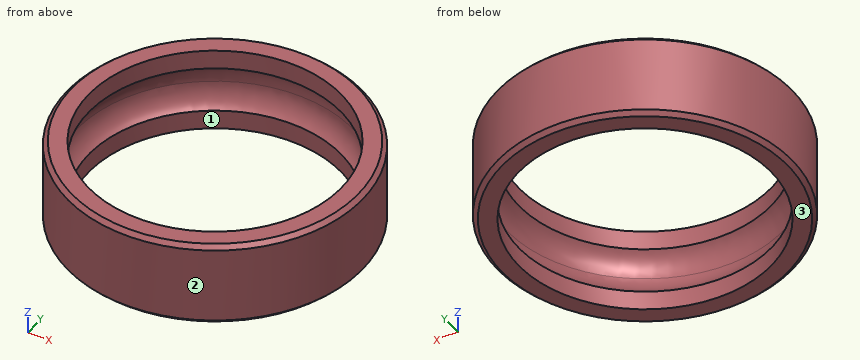
Solid Edge part; units mm, degrees
sketch "Sketch1" plane through (0, 0, 0) normal (0, -1, 0) x (1, 0, 0)
  line L0 (30, -10) -> (30, 10)
  line L1 (30, 10) -> (35, 10)
  line L2 (35, 10) -> (35, -10)
  line L3 (35, -10) -> (30, -10)
  dimension "D1" = 30
  dimension "D2" = 35
revolve "RevolvedProtrusion1" add sketch "Sketch1" angle 360 about axis through (0, 0, 54) along (0, 0, -1)
sketch "Sketch2" plane through (0, 0, 0) normal (0, -1, 0) x (1, 0, 0)
  circle A0 centre (26, 0) radius 6.75
revolve "RevolvedCutout1" cut sketch "Sketch2" angle 360 about axis through (0, 0, 54) along (0, 0, -1)
chamfer "Chamfer1" distance 1 angle 45 2 edges at (-35, 0, 10) (-35, 0, -10)
properties material "Polyethylene, low density"
Check sheet for the modelled part. Datum: model origin and axes. Units: mm. Face numbers are marked on the shaded views. Coordinates: 2 decimals unless noted, no trailing zeros. Loops run counter-clockwise (first coordinate to the right, second up) from the corner with the lowest first, then second, coordinate; pieces in that order, holes last.
1) Gauge pin test, flat ends, axial feed: pin 1 (12 mm diameter, centred on x = -13, z = -8, fed in from -Y); pin 2 (8 mm diameter, centred on x = -15.5, z = 6.5, fed in from -Y); pin 3 (6 mm diameter, centred on y = -2, z = 1, fed in from -X); pin 4 (8 mm diameter, centred on x = -3, z = 0, fed in from +Y). Record the tip position at first contact, or that the pin passes through.
2) Sectioned sample at A-A (x = 0). Record the boundary of the cut face in (y, z).
3) Sectioned sample at D-D (z = 1.25). Record the boundary of the cut face in (x, y), and give its area (3 significant figures).
4) Material ranges on probe 1 along Y at (x, z) = (0, -8.05); probe 2 along X at (y, z) = (-11.5, -6.75), recorded low to high.
5) Sectioned sample at C-C (z = 7.25). Record the boundary of the cut face in (x, y), and give its area (3 significant figures).
6) Release check for a two-part mould opening along X. For the marked faces 1, 2 and 3 record: released by +X, released by -X, zero draft, split by the parting line, or undercut.
Check sheet entries:
1. pin 1: stops at y = -34.29
1. pin 2: stops at y = -33.06
1. pin 3: stops at x = -35
1. pin 4: stops at y = 35
2. outline: (-35, -9) - (-34, -10) - (-30, -10) - (-30, -5.44) arc R6.75 cw to (-30, 5.44) - (-30, 10) - (-34, 10) - (-35, 9) - close; (30, -10) - (34, -10) - (35, -9) - (35, 9) - (34, 10) - (30, 10) - (30, 5.44) arc R6.75 cw to (30, -5.44) - close
3. outline: circle Ø70 at (0, 0); hole circle Ø65.27 at (0, 0)
3. area: 503 mm2
4. probe 1: y = -35 to -30, 30 to 35
4. probe 2: x = -33.06 to -27.71, 27.71 to 33.06
5. outline: circle Ø70 at (0, 0); hole circle Ø60 at (0, 0)
5. area: 1,020 mm2
6. face 1: undercut
6. face 2: split by the parting line
6. face 3: zero draft
